```python
from build123d import *

# Parameters (mm, degrees)
F0_W     = 152.4
F0_H     = 76.2
F1_DEPTH = 101.6
F2_W     = 50.8
F2_H     = 50.8
F3_DEPTH = 50.8
F4_DEPTH = 50.8


with BuildPart() as f1:
    # F0 (on Top) → F1 (new body)
    with BuildSketch(Plane.XY):
        with Locations((15.3874829412, -8.4786337945)):
            Rectangle(F0_W, F0_H)
    extrude(amount=F1_DEPTH)

    # F2 (on face) → F3 (cut)
    with BuildSketch(Plane.XZ.offset(46.5786337945)):
        with Locations((-35.4125170588, 76.2)):
            Rectangle(F2_W, F2_H)
    extrude(amount=-F3_DEPTH, mode=Mode.SUBTRACT)

    # F2 (on face) → F4 (cut)
    with BuildSketch(Plane.XZ.offset(46.5786337945)):
        with Locations((66.1874829412, 76.2)):
            Rectangle(F2_W, F2_H)
    extrude(amount=-F4_DEPTH, mode=Mode.SUBTRACT)


solid = f1.part
```
Source: CAD feature listing. Evaluate the final solid. Frame: model axes, mm. A direction names the side the tool comes from. Coordinates: 2 decimals unless noted, no trailing zeros. Write each loop counter-clockwise with the first axis right and the second up, starting at its lowest first coordinate (ties: lowest second). Pieces come first, ordered by that corner, then holes. Notation, with made-up numbers: (-24, 25.25) -> (-19, 25.25) arc R25 cw to (-19, 43.25) -> close; hole circle Ø1 at (61.5, 23.5). An arc over 180 degrees is marked (long way). Return JSON: item names as keys, results as strings. Group by question number.
1) Ray query, line 1 along Y through (x, z) = (66.5, 85); line 2 along Z through (x, y) = (-20, -4); line 3 along X through (y, z) = (-24.5, 70). Return the intervals inside material, ascending.
2) Section query B-B, the plane y = -26. Return loops of the section in (x, z).
3) Section query C-C, the plane x = -13.5. Return loops of the section in (y, z), plus the area to 3 significant figures.
4) Section query A-A, the plane z = 59. Return loops of the section in (x, y), plus the area to 3 significant figures.
5) Contact query for flat-ended pins moving along their axis: P1, Ø10, axis at y = -2.5, z = 84, coming from the +X side; P2, Ø8, axis at x = 60.5, z = 76.5, coming from the -Y side. Output: stop coordinate, or through.
6) Set-up query: faces 1 (the face through (14, -8, 0)), 2 (the face through (40.787, -22, 76)), 3 (the face through (-36, 4.221, 77)). Return all of +Z, -Z, +X, -X, +Y, -Y with unobstructed straight access to the full face (end or side cutting, diameter ignored); none if empty.
From the geometry:
{
 "1": {"line 1": "4.22 to 29.62", "line 2": "0 to 50.8", "line 3": "-10.01 to 40.79"},
 "2": {"outline": "(-60.81, 0) -> (91.59, 0) -> (91.59, 50.8) -> (40.79, 50.8) -> (40.79, 101.6) -> (-10.01, 101.6) -> (-10.01, 50.8) -> (-60.81, 50.8) -> close"},
 "3": {"outline": "(-46.58, 0) -> (29.62, 0) -> (29.62, 101.6) -> (4.22, 101.6) -> (4.22, 50.8) -> (-46.58, 50.8) -> close", "area": "5,160 mm²"},
 "4": {"outline": "(-60.81, 4.22) -> (-10.01, 4.22) -> (-10.01, -46.58) -> (40.79, -46.58) -> (40.79, 4.22) -> (91.59, 4.22) -> (91.59, 29.62) -> (-60.81, 29.62) -> close", "area": "6,450 mm²"},
 "5": {"P1": "x = 40.79", "P2": "y = 4.22"},
 "6": {"face 1": "-Z, +X, -X, +Y, -Y", "face 2": "+Z, +X, -Y", "face 3": "+Z, -X, -Y"}
}
